from build123d import *

# Parameters (mm, degrees)
SKETCH3_R           = 26.878
SKETCH3_R_2         = 26.128
BOSS_EXTRUDE1_DEPTH = 10
SKETCH5_R           = 1.5
BOSS_EXTRUDE4_DEPTH = 5.5
CUT_EXTRUDE1_DEPTH  = 3.5
BOSS_EXTRUDE5_START = -3.5
SKETCH8_R           = 26.128
SKETCH8_R_2         = 25.5
BOSS_EXTRUDE5_DEPTH = 1.5


with BuildPart() as part:
    # Sketch3 → Boss-Extrude1 (new body)
    with BuildSketch(Plane(origin=(0, 0, 0), x_dir=(1, 0, 0), z_dir=(0, 1, 0))):
        with Locations(Location((0, 0, 0), (0, 0, 270))):
            Circle(SKETCH3_R)
        with Locations(Location((0, 0, 0), (0, 0, 270))):
            Circle(SKETCH3_R_2, mode=Mode.SUBTRACT)
    extrude(amount=BOSS_EXTRUDE1_DEPTH)

    # Sketch5 → Boss-Extrude4 (add)
    with BuildSketch(Plane.XZ):
        with BuildLine():
            Line((-5.543162198, -29.995394675), (-5.543162198, -26.300194616))
            ThreePointArc((-5.543162198, -26.300194616), (-0.534858171, -26.863033142), (4.491880525, -26.499997988))
            Line((4.491880525, -26.499997988), (4.491880525, -29.995394675))
            ThreePointArc((4.491880525, -29.995394675), (-0.525640836, -35.012916036), (-5.543162198, -29.995394675))
        make_face()
        with Locations(Location((-0.525640836, -29.995394675, 0), (0, 0, 270))):
            Circle(SKETCH5_R, mode=Mode.SUBTRACT)
    extrude(amount=-BOSS_EXTRUDE4_DEPTH)

    # Sketch6 → Cut-Extrude1 (cut)
    with BuildSketch(Plane(origin=(0, 0, 0), x_dir=(-1, 0, 0), z_dir=(0, -1, 0))):
        with BuildLine():
            Line((4.710133197, 29.995394675), (4.710133197, 25.699942204))
            ThreePointArc((4.710133197, 25.699942204), (0.530383369, 26.096098926), (-3.658851524, 25.81760336))
            Line((-3.658851524, 25.81760336), (-3.658851524, 29.995394675))
            ThreePointArc((-3.658851524, 29.995394675), (0.525640836, 34.179887036), (4.710133197, 29.995394675))
        make_face()
    extrude(amount=-CUT_EXTRUDE1_DEPTH, mode=Mode.SUBTRACT)

    # Sketch7 → Revolve1 (revolve)
    with BuildSketch(Plane.XY, mode=Mode.PRIVATE) as revolve1_sk:
        Polygon((-26.878, 10), (-14.897981914, 30.75), (-10.897981914, 30.75), (-10.897981914, 30), (-14.580994616, 30), (-26.128, 10), align=None)
    revolve(revolve1_sk.sketch.rotate(Axis((0, 30.1875, 0), (0, -1, 0)), 270), axis=Axis((0, 30.1875, 0), (0, -1, 0)))

    # Sketch8 → Boss-Extrude5 (add)
    with BuildSketch(Plane.XZ.offset(BOSS_EXTRUDE5_START)):
        with Locations(Location((0, 0, 0), (0, 0, 270))):
            Circle(SKETCH8_R)
        with Locations(Location((0, 0, 0), (0, 0, 270))):
            Circle(SKETCH8_R_2, mode=Mode.SUBTRACT)
    extrude(amount=-BOSS_EXTRUDE5_DEPTH)


solid = part.part
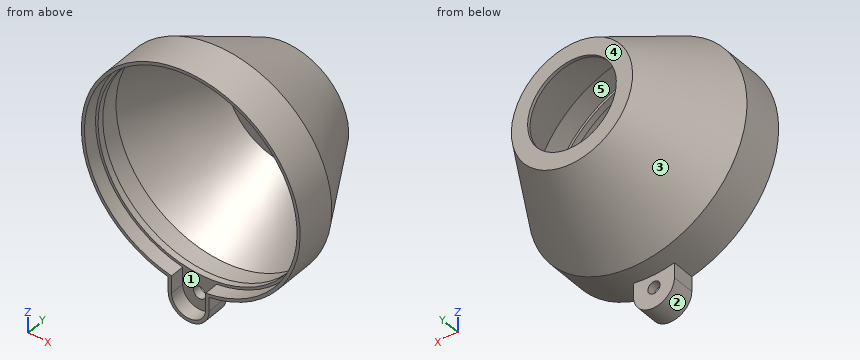
Verification items for the finished model (mm, model axes). Face numbers are marked on the shaded views. A direction names the side the tool comes from. Round coordinates to 2 decimals unless told otherwise and drop trailing zeros. Write each loop counter-clockwise with the first axis right and the second up, starting at its lowest first coordinate (ties: lowest second). Pieces come first, ordered by that corner, then holes.
(1) Section check B-B (y = 9). Enter the section's corners in (x, z).
Returned:
outline: circle Ø53.76 at (0, 0); hole circle Ø52.26 at (0, 0)
(2) Access from +Z, -Z, +X, -X, +Y, -Y to the whole of each face (thin tool, end or side, straight path). Record for the marked faces 1 and 2.
Returned:
face 1: -Y
face 2: -Z, +Y, -Y
(3) Mould release check, pull along Z, two halves, no side actions. Record for the marked faces 3, 4 and 5: pulls with the +Z half, pulls with the -Z half, needs draft (parallel to the pull), parting line crosses it, or undercut.
Returned:
face 3: parting line crosses it
face 4: needs draft
face 5: undercut
(4) Section check A-A (z = 0). Enter the section's corners in (x, y).
Returned:
outline: (-26.88, 0) - (-26.13, 0) - (-26.13, 3.5) - (-25.5, 3.5) - (-25.5, 5) - (-26.13, 5) - (-26.13, 10) - (-14.58, 30) - (-10.9, 30) - (-10.9, 30.75) - (-14.9, 30.75) - (-26.88, 10) - close; (10.9, 30) - (14.58, 30) - (26.13, 10) - (26.13, 5) - (25.5, 5) - (25.5, 3.5) - (26.13, 3.5) - (26.13, 0) - (26.88, 0) - (26.88, 10) - (14.9, 30.75) - (10.9, 30.75) - close
(5) Material ranges on line 1 (X direction, y = 3.95, z = 0); line 2 (X direction, y = 5.5, z = -0.5); line 3 (Z direction, x = -10, y = 11.5), recorded low to high.
Returned:
line 1: x = -26.88 to -25.5, 25.5 to 26.88
line 2: x = -26.87 to -26.12, 26.12 to 26.87
line 3: z = -24.01 to -23.2, 23.2 to 24.01
(6) Section check C-C (y = 14.5). Enter the section's corners in (x, z), plus the area to 3 significant figures.
Returned:
outline: circle Ø48.56 at (0, 0); hole circle Ø47.06 at (0, 0)
area: 113 mm2
(7) Depth check by flat-ended pin: pin 1 Ø1 at (y, z) = (3, -29) entering from +X; pin 2 Ø23.5 at (x, z) = (-3, -4.5) entering from -Y; pin 3 Ø2 at (x, y) = (-5.5, 11.5) entering from +Z; pin 4 Ø2.5 at (x, z) = (-0.53, -30) entering from +Y. Enter the tip coordinate at first touch or a pass-through.
Returned:
pin 1: stops at x = 4.49
pin 2: stops at y = 25.54
pin 3: stops at z = 26.05
pin 4: passes through
